Geometry check sheet. Reference: drawing and pictorial views, mm from the part's lowest x, y, z. A direction names the side the tool comes from. Give positions to 0.01 mm unless a question says otherwise; leave off trailing zeros. Write each loop counter-clockwise with the first axis right and the second up, starting at its lowest first coordinate (ties: lowest second). Pieces come first, ordered by that corner, then holes. Notation, with made-up numbers: (37.25, 40) -> (62.25, 40) arc R21 cw to (62.25, 46) -> close; hole circle Ø8 at (21, -17.5). An arc over 180 degrees is marked (long way). Use a Markdown table: item, result. Add a question column.
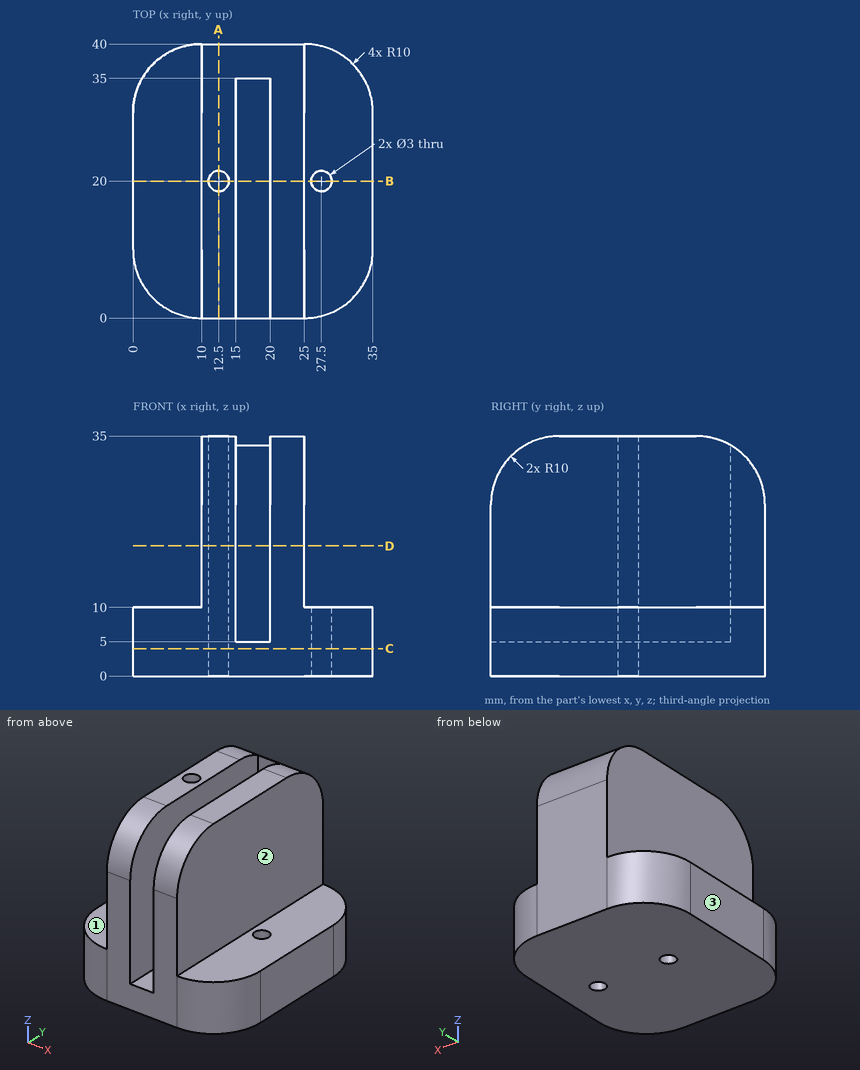
1) Gauge pin test, flat ends, axial feed: P1, Ø3, axis at y = 17, z = 29, coming from the -X side; P2, Ø1.5, axis at x = 17, z = 19, coming from the -Y side; P3, Ø1.5, axis at y = 32.5, z = 27, coming from the +X side. Record the tip position at first contact, or that the pin passes through.
2) Sectioned sample at C-C, the plane z = 4. Enter the section's corners in (x, y), and give its area (3 significant figures).
3) Sectioned sample at A-A, the plane x = 12.5. Enter the section's corners in (y, z).
4) Tool access check on the marked faces 1, 2 and 3. Record the directions out of +Z, -Z, +X, -X, +Y, -Y that give a thin tool (end or side, any length) a straight path to the whole face; none if there is none.
5) Sectioned sample at B-B, the plane y = 20. Enter the section's corners in (x, z).
6) Material ranges on probe 1 along X at (y, z) = (20, 24); probe 2 along X at (y, z) = (20, 8); probe 3 along X at (y, z) = (19.5, 11), recorded low to high. Write a range as [from, to].
7) Sectioned sample at D-D, the plane z = 19. Enter the section's corners in (x, y), and give its area (3 significant figures).
Check values:
| question | item | result |
|---|---|---|
| 1 | P1 | x = 10 |
| 1 | P2 | y = 35 |
| 1 | P3 | x = 25 |
| 2 | outline | (0, 10) arc R10 ccw to (10, 0) -> (25, 0) arc R10 ccw to (35, 10) -> (35, 30) arc R10 ccw to (25, 40) -> (10, 40) arc R10 ccw to (0, 30) -> close; hole circle Ø3 at (12.5, 20); hole circle Ø3 at (27.5, 20) |
| 2 | area | 1,300 mm² |
| 3 | outline | (0, 0) -> (18.5, 0) -> (18.5, 35) -> (10, 35) arc R10 ccw to (0, 25) -> close; (21.5, 0) -> (40, 0) -> (40, 25) arc R10 ccw to (30, 35) -> (21.5, 35) -> close |
| 4 | face 1 | +Z, -X, +Y, -Y |
| 4 | face 2 | +Z, +X, +Y, -Y |
| 4 | face 3 | +Z, -Z, -X, +Y, -Y |
| 5 | outline | (0, 0) -> (11, 0) -> (11, 35) -> (10, 35) -> (10, 10) -> (0, 10) -> close; (14, 0) -> (26, 0) -> (26, 10) -> (25, 10) -> (25, 35) -> (20, 35) -> (20, 5) -> (15, 5) -> (15, 35) -> (14, 35) -> close; (29, 0) -> (35, 0) -> (35, 10) -> (29, 10) -> close |
| 6 | probe 1 | [10, 11], [14, 15], [20, 25] |
| 6 | probe 2 | [0, 11], [14, 15], [20, 26], [29, 35] |
| 6 | probe 3 | [10, 11.09], [13.91, 15], [20, 25] |
| 7 | outline | (10, 0) -> (15, 0) -> (15, 35) -> (20, 35) -> (20, 0) -> (25, 0) -> (25, 40) -> (10, 40) -> close; hole circle Ø3 at (12.5, 20) |
| 7 | area | 418 mm² |
